```python
from build123d import *

# Parameters (mm, degrees)
SKETCH2_W           = 50.5
SKETCH2_H           = 40.5
SKETCH2_W_2         = 20.5
SKETCH2_H_2         = 20.5
BOSS_EXTRUDE3_DEPTH = 25
BOSS_EXTRUDE5_DEPTH = 30
SKETCH6_W           = 50.5
SKETCH6_H           = 40.5
SKETCH6_W_2         = 20.5
SKETCH6_H_2         = 20.5
BOSS_EXTRUDE6_DEPTH = 25
FILLET6_R           = 5
FILLET8_R           = 5
FILLET10_R          = 5
HOLE1_OUTLINE_R     = 2.5
HOLE1_DEPTH         = 40.5
HOLE2_OUTLINE_R     = 2.5
HOLE2_DEPTH         = 40.5
FILLET11_R          = 5


# Read off the part's stored shape, not the designer's step: Hole1, Hole2
with BuildPart() as part:
    # Sketch2 → Boss-Extrude3 (new body)
    with BuildSketch(Plane.XY):
        with Locations((25.25, 20.25)):
            Rectangle(SKETCH2_W, SKETCH2_H)
        with Locations((20.25, 20.25)):
            Rectangle(SKETCH2_W_2, SKETCH2_H_2, mode=Mode.SUBTRACT)
    extrude(amount=BOSS_EXTRUDE3_DEPTH)

    # Sketch5 → Boss-Extrude5 (add)
    with BuildSketch(Plane.XY.offset(25)):
        Polygon((50.5, 40.5), (50.5, 0), (50.5, -5), (30.5, -5), (30.5, 0), (30.5, 5), (35.5, 5), (35.5, 35.5), (30.5, 35.5), (30.5, 40.5), (30.5, 45.5), (50.5, 45.5), align=None)
    extrude(amount=BOSS_EXTRUDE5_DEPTH)

    # Sketch6 → Boss-Extrude6 (add)
    with BuildSketch(Plane.XY.offset(55)):
        with Locations((25.25, 20.25)):
            Rectangle(SKETCH6_W, SKETCH6_H)
        with Locations((20.25, 20.25)):
            Rectangle(SKETCH6_W_2, SKETCH6_H_2, mode=Mode.SUBTRACT)
    extrude(amount=BOSS_EXTRUDE6_DEPTH)

    # Fillet6
    fillet6_edges = [part.edges().sort_by_distance(p)[0] for p in [
        (50.5, 0, 67.5),
        (50.5, 40.5, 67.5),
        (50.5, 40.5, 12.5),
        (50.5, 0, 12.5),
    ]]
    fillet(fillet6_edges, radius=FILLET6_R)

    # Fillet8
    fillet8_edges = [part.edges().sort_by_distance(p)[0] for p in [
        (22.75, 0, 0),
        (22.75, 0, 80),
        (50.5, 20.25, 0),
        (50.5, 20.25, 80),
        (22.75, 40.5, 80),
        (49.035533906, 39.035533906, 80),
        (49.035533906, 1.464466094, 80),
        (22.75, 40.5, 0),
        (49.035533906, 39.035533906, 0),
        (49.035533906, 1.464466094, 0),
    ]]
    fillet(fillet8_edges, radius=FILLET8_R)

    # Fillet10
    # the kernel refuses this fillet: 5 mm, written as the material it takes off along each edge
    with BuildSketch(Plane(origin=(-12.5, 0, 25), x_dir=(0, 0, -1), z_dir=(1, 0, 0)), Plane(origin=(-12.5, 0, 55), x_dir=(0, 1, 0), z_dir=(1, 0, 0)), Plane(origin=(30.5, 40.5, 55), x_dir=(0, -1, 0), z_dir=(-1, 0, 0))) as fillet10_piece_1:
        with BuildLine():
            CenterArc((FILLET10_R, FILLET10_R), FILLET10_R, 180, 90)
            Line((0, FILLET10_R), (0, 0))
            Line((0, 0), (FILLET10_R, 0))
        make_face()
    extrude(amount=43, mode=Mode.SUBTRACT)
    with BuildSketch(Plane(origin=(30.5, 40.5, 25), x_dir=(0, -1, 0), z_dir=(-1, 0, 0))) as fillet10_piece_2:
        with BuildLine():
            CenterArc((FILLET10_R, -FILLET10_R), FILLET10_R, 90, 90)
            Line((0, -FILLET10_R), (0, 0))
            Line((0, 0), (FILLET10_R, 0))
        make_face()
    extrude(amount=43, mode=Mode.SUBTRACT)

    # Hole1 outline → Hole1 (cut)
    with BuildSketch(Plane(origin=(0, 0, 0), x_dir=(1, 0, 0), z_dir=(0, 1, 0))):
        with Locations((20, -67.5)):
            Circle(HOLE1_OUTLINE_R)
    extrude(amount=HOLE1_DEPTH, mode=Mode.SUBTRACT)

    # Hole2 outline → Hole2 (cut)
    with BuildSketch(Plane(origin=(0, 0, 0), x_dir=(1, 0, 0), z_dir=(0, 1, 0))):
        with Locations((20, -12.5)):
            Circle(HOLE2_OUTLINE_R)
    extrude(amount=HOLE2_DEPTH, mode=Mode.SUBTRACT)

    # Fillet11
    fillet11_edges = [part.edges().sort_by_distance(p)[0] for p in [
        (30.5, -5, 40),
        (30.5, 45.5, 40),
    ]]
    fillet(fillet11_edges, radius=FILLET11_R)


solid = part.part
```
Geometry: final body of the model. Coordinates: model frame, mm. A direction names the side the tool comes from. Round coordinates to 2 decimals unless told otherwise and drop trailing zeros. Loops run counter-clockwise (first coordinate to the right, second up) from the corner with the lowest first, then second, coordinate; pieces in that order, holes last. Notation, with made-up numbers: (-25, 3.25) -> (25, 3.25) arc R20 cw to (25, 8.25) -> close; hole circle Ø4 at (55.25, -6.75). An arc over 180 degrees is marked (long way). Use one line per item in the form item = value.
Item 1: Access query for faces 1 (the cylindrical face through (15.46, 39.07, 56.5)), 2 (the flat face through (35.5, 20, 40)), 3 (the flat face through (22, 40.5, 65)), 4 (the flat face through (30.5, 20, 67)). Directions: +Z, -Z, +X, -X, +Y, -Y. A direction counts if a zero-diameter tool reaches every point of the face in a straight line with its end or side. Return the directions, or none.
Evaluation:
face_1 = -X, +Y
face_2 = -X
face_3 = +Z, +X, -X, +Y
face_4 = +Z, -Z
Item 2: Cut plane A-A on x = 9. Output: boundary loops of the cut face in (y, z).
Evaluation:
outline = (0, 5) arc R5 ccw to (5, 0) -> (35.5, 0) arc R5 ccw to (40.5, 5) -> (40.5, 20) arc R5 ccw to (35.5, 25) -> (5, 25) arc R5 ccw to (0, 20) -> close; (0, 60) arc R5 ccw to (5, 55) -> (35.5, 55) arc R5 ccw to (40.5, 60) -> (40.5, 75) arc R5 ccw to (35.5, 80) -> (5, 80) arc R5 ccw to (0, 75) -> close
Item 3: Material intervals for probe 1 along Y at (x, z) = (21.5, 5.5); probe 2 along X at (y, z) = (33.75, 67.5); probe 3 along X at (y, z) = (21, 11), sorted ascending.
Evaluation:
probe_1 = 0 to 10, 30.5 to 40.5
probe_2 = 0 to 17.5, 22.5 to 50.5
probe_3 = 0 to 10, 30.5 to 50.5
Item 4: Draft query along Y for faces 5 (the flat face through (50.5, 20, 40)), 6 (the flat face through (20.1, 30.5, 9.5)), 7 (the flat face through (22, 40.5, 15)). Return one class per face: released by +Y, released by -Y, zero draft, split by the parting line, or undercut.
Evaluation:
face_5 = zero draft
face_6 = undercut
face_7 = released by +Y
Item 5: Cut plane B-B on y = 9. Output: boundary loops of the cut face in (x, z), then the cut area to 4 significant figures.
Evaluation:
outline = (0, 0) -> (45.5, 0) arc R5 ccw to (50.5, 5) -> (50.5, 75) arc R5 ccw to (45.5, 80) -> (0, 80) -> (0, 55) -> (35.5, 55) -> (35.5, 25) -> (0, 25) -> close; hole circle Ø5 at (20, 12.5); hole circle Ø5 at (20, 67.5)
area = 2,925 mm2
Item 6: Contact query for flat-ended pins moving along their axis: pin 1 Ø1.5 at (x, z) = (36.5, 66) entering from +Y; pin 2 Ø8 at (x, z) = (17, 60.5) entering from -Y; pin 3 Ø11 at (x, y) = (39.5, -1.5) entering from +Z; pin 4 Ø4 at (x, z) = (20, 67.5) entering from -Y. Output: stop coordinate, or through.
Evaluation:
pin_1 = 40.5
pin_2 = 0
pin_3 = 79.9
pin_4 = through
Item 7: Cut plane D-D on y = 28.5. Output: boundary loops of the cut face in (x, z), then the cut area to 3 significant figures.
Evaluation:
outline = (0, 0) -> (10, 0) -> (10, 25) -> (0, 25) -> close; (0, 55) -> (10, 55) -> (10, 80) -> (0, 80) -> close; (30.5, 0) -> (45.5, 0) arc R5 ccw to (50.5, 5) -> (50.5, 75) arc R5 ccw to (45.5, 80) -> (30.5, 80) -> (30.5, 55) -> (35.5, 55) -> (35.5, 25) -> (30.5, 25) -> close
area = 1,940 mm2
Item 8: Cut plane C-C on z = 12.5. Output: boundary loops of the cut face in (x, y).
Evaluation:
outline = (0, 0) -> (17.5, 0) -> (17.5, 10) -> (10, 10) -> (10, 30.5) -> (17.5, 30.5) -> (17.5, 40.5) -> (0, 40.5) -> close; (22.5, 0) -> (45.5, 0) arc R5 ccw to (50.5, 5) -> (50.5, 35.5) arc R5 ccw to (45.5, 40.5) -> (22.5, 40.5) -> (22.5, 30.5) -> (30.5, 30.5) -> (30.5, 10) -> (22.5, 10) -> close
